from build123d import *

# Parameters (mm, degrees)
SKETCH_1_W          = 15.8
SKETCH_1_H          = 7.8
SKETCH_1_R          = 2.4
EXTRUDE_1_DEPTH     = 3.2
SKETCH_2_R          = 2.4
SKETCH_2_R_2        = 1.6
EXTRUDE_2_DEPTH     = 1.7
SKETCH_3_R          = 2.5
CUT_EXTRUDE_1_DEPTH = 1.8


with BuildPart() as part:
    # Эскиз1 → Бобышка-Вытянуть1 (new body)
    # profile 1 of 2: a face of its own
    with BuildSketch(Plane(origin=(0, 0, 0), x_dir=(1, 0, 0), z_dir=(0, 1, 0))):
        Rectangle(SKETCH_1_W, SKETCH_1_H)
        Circle(SKETCH_1_R, mode=Mode.SUBTRACT)
    # profile 2 of 2: a face of its own
    with BuildSketch(Plane(origin=(0, 0, 0), x_dir=(1, 0, 0), z_dir=(0, 1, 0))):
        Circle(SKETCH_1_R)
    extrude(amount=EXTRUDE_1_DEPTH)

    # Эскиз2 → Бобышка-Вытянуть2 (add)
    with BuildSketch(Plane(origin=(0, 0, 0), x_dir=(1, 0, 0), z_dir=(0, 1, 0))):
        with Locations(Location((0, 0, 0), (0, 0, 270))):
            Circle(SKETCH_2_R)
        with Locations(Location((0, 0, 0), (0, 0, 270))):
            Circle(SKETCH_2_R_2, mode=Mode.SUBTRACT)
    extrude(amount=-EXTRUDE_2_DEPTH)

    # Эскиз3 → Вырез-Вытянуть1 (cut)
    with BuildSketch(Plane(origin=(0, 3.2, 0), x_dir=(1, 0, 0), z_dir=(0, 1, 0))):
        with Locations(Location((0, 0, 0), (0, 0, 270))):
            Circle(SKETCH_3_R)
    extrude(amount=-CUT_EXTRUDE_1_DEPTH, mode=Mode.SUBTRACT)


solid = part.part
The listing builds one solid part. Answer for the finished solid, in the listing's coordinates (mm). A direction names the side the tool comes from. Coordinates: 2 decimals unless noted, no trailing zeros. Write each loop counter-clockwise with the first axis right and the second up, starting at its lowest first coordinate (ties: lowest second). Pieces come first, ordered by that corner, then holes. Notation, with made-up numbers: (36.25, 80.5) - (45.25, 80.5) arc R9 cw to (45.25, 84.5) - close; hole circle Ø3 at (59, 9). An arc over 180 degrees is marked (long way). Return JSON: item names as keys, results as strings.
1. The part is cut by section B-B on x = 0. Determine the outline of the cut face in (y, z), then the cut area to 3 significant figures.
Final values:
{"outline": "(-1.7, -2.4) - (0, -2.4) - (0, -3.9) - (3.2, -3.9) - (3.2, -2.5) - (1.4, -2.5) - (1.4, 2.5) - (3.2, 2.5) - (3.2, 3.9) - (0, 3.9) - (0, 2.4) - (-1.7, 2.4) - (-1.7, 1.6) - (0, 1.6) - (0, -1.6) - (-1.7, -1.6) - close", "area": "18.7 mm^2"}
2. The part is cut by section A-A on z = 0. Determine the outline of the cut face in (x, y), then the cut area to 3 significant figures.
Final values:
{"outline": "(-7.9, 0) - (-2.4, 0) - (-2.4, -1.7) - (-1.6, -1.7) - (-1.6, 0) - (1.6, 0) - (1.6, -1.7) - (2.4, -1.7) - (2.4, 0) - (7.9, 0) - (7.9, 3.2) - (2.5, 3.2) - (2.5, 1.4) - (-2.5, 1.4) - (-2.5, 3.2) - (-7.9, 3.2) - close", "area": "44.3 mm^2"}
3. For a pull along Z with two mould halves and no side action, classify faces 1 (the face through (2.024, -0.838, 1.29)), 2 (the face through (0, 0, 0)), 3 (the face through (7.9, 2, 0)), 4 (the face through (0, 2, -3.9)) as +Z half, -Z half, draft (parallel to the pull), parting line (faces both ways), or undercut.
Final values:
{"face 1": "parting line", "face 2": "undercut", "face 3": "draft", "face 4": "-Z half"}
4. The part is cut by section C-C on y = -0.3. Determine the outline of the cut face in (x, z).
Final values:
{"outline": "circle Ø4.8 at (0, 0); hole circle Ø3.2 at (0, 0)"}
5. Which of the six approach directions +Z, -Z, +X, -X, +Y, -Y give full straight-line access (tool end or side, diameter ignored) to faces 5 (the face through (-2, -1.7, 0)), 6 (the face through (-2.44, 2.31, -0.54)), 7 (the face through (-0.97, -0.84, -1.27))?
Final values:
{"face 5": "+Z, -Z, +X, -X, -Y", "face 6": "+Y", "face 7": "-Y"}
6. This flat-tipped pin is pushed along its axis until it touches: pin 1 Ø2.5 at (x, z) = (-3.5, 1.5) entering from -Y. Where does it stop, or does it pass through?
Final values:
{"pin 1": "y = 0"}
7. The part is cut by section D-D on z = 2.25. Determine the outline of the cut face in (x, y).
Final values:
{"outline": "(-7.9, 0) - (-0.84, 0) - (-0.84, -1.7) - (0.84, -1.7) - (0.84, 0) - (7.9, 0) - (7.9, 3.2) - (1.09, 3.2) - (1.09, 1.4) - (-1.09, 1.4) - (-1.09, 3.2) - (-7.9, 3.2) - close"}
8. Consider line 1 along X through (y, z) = (-0.8, 0); line 2 along Y through (x, z) = (3, -0.5); line 3 along Z through (x, y) = (0.25, 1.9). Determine where each line is inside the solid, lowest interval first.
Final values:
{"line 1": "-2.4 to -1.6, 1.6 to 2.4", "line 2": "0 to 3.2", "line 3": "-3.9 to -2.49, 2.49 to 3.9"}
